from build123d import *

# Parameters (mm, degrees)
SKICA1_W                = 18.57
SKICA1_H                = 8.22
P_IDAT_VYSUNUT_M1_DEPTH = 5
SKICA2_W                = 18.7
SKICA2_H                = 4.88
P_IDAT_VYSUNUT_M2_DEPTH = 28.3
SKICA3_W                = 13.3
SKICA3_H                = 1.1
P_IDAT_VYSUNUT_M3_DEPTH = 5.3


with BuildPart() as part:
    # Skica1 → Přidat vysunutím1 (new body)
    with BuildSketch(Plane.XY):
        Rectangle(SKICA1_W, SKICA1_H)
    extrude(amount=P_IDAT_VYSUNUT_M1_DEPTH)

    # Skica2 → Přidat vysunutím2 (add)
    with BuildSketch(Plane(origin=(0, 4.11, 0), x_dir=(1, 0, 0), z_dir=(0, 1, 0))):
        with Locations((0, -2.5)):
            Rectangle(SKICA2_W, SKICA2_H)
    extrude(amount=P_IDAT_VYSUNUT_M2_DEPTH)

    # Skica3 → Přidat vysunutím3 (add)
    with BuildSketch(Plane(origin=(0, 32.41, 0), x_dir=(1, 0, 0), z_dir=(0, 1, 0))):
        with Locations((0, -4.39)):
            Rectangle(SKICA3_W, SKICA3_H)
    extrude(amount=P_IDAT_VYSUNUT_M3_DEPTH)


solid = part.part
Build history of the part. All positions in model axes, mm. A direction names the side the tool comes from. Coordinates: 2 decimals unless noted, no trailing zeros. Order: outer loops, then holes, each group sorted by start corner. A loop starts at its lowest first (then second) coordinate and runs counter-clockwise, first axis right, second up. Notation, with made-up numbers: (70, 10) - (129, 10) arc R15 cw to (129, 19) - close; hole circle Ø11 at (-12, 16). An arc over 180 degrees is marked (long way). Write item = value, one per line. Start each with the question number.
1) Saw through at A-A on z = 1.1. Write the cut outline in (x, y) (3 decimals), then the cut area to 3 significant figures.
2) Flat gauge pins, fed straight in: pin 1 Ø9.5 at (x, y) = (-4.5, 18) entering from -Z; pin 2 Ø1.2 at (y, z) = (35.5, 4.5) entering from +X; pin 3 Ø2.5 at (x, y) = (3.5, 35) entering from -Z. Where does each tip first touch, or does it go through?
3) Saw through at D-D on z = 4.35. Write the cut outline in (x, y) (3 decimals).
4) Saw through at C-C on y = 6.5. Write the cut outline in (x, z).
5) Saw through at B-B on x = -7.25. Write the cut outline in (y, z).
6) 3-axis set-ups, long thin cutter, end or side, ignore diameter. For faces 1 (the face through (-6.65, 35, 4)), 2 (the face through (6.65, 35, 4)), 3 (the face through (0, 21, 4.94)): which of +Z, -Z, +X, -X, +Y, -Y reach the whole face in a straight line?
7) Wall check: line 1 along Y through (x, z) = (-8, 4.3); line 2 along Z through (x, y) = (-5, 11). Give the ranges that are in metal, low to high. Write a range as from..to.
From the geometry:
q1.outline = (-9.35, 4.11) - (-9.285, 4.11) - (-9.285, -4.11) - (9.285, -4.11) - (9.285, 4.11) - (9.35, 4.11) - (9.35, 32.41) - (-9.35, 32.41) - close
q1.area = 682 mm^2
q2.pin_1 = 0.06
q2.pin_2 = 6.65
q2.pin_3 = 3.84
q3.outline = (-9.35, 4.11) - (-9.285, 4.11) - (-9.285, -4.11) - (9.285, -4.11) - (9.285, 4.11) - (9.35, 4.11) - (9.35, 32.41) - (6.65, 32.41) - (6.65, 37.71) - (-6.65, 37.71) - (-6.65, 32.41) - (-9.35, 32.41) - close
q4.outline = (-9.35, 0.06) - (9.35, 0.06) - (9.35, 4.94) - (-9.35, 4.94) - close
q5.outline = (-4.11, 0) - (4.11, 0) - (4.11, 0.06) - (32.41, 0.06) - (32.41, 4.94) - (4.11, 4.94) - (4.11, 5) - (-4.11, 5) - close
q6.face_1 = +Z, -Z, -X, +Y
q6.face_2 = +Z, -Z, +X, +Y
q6.face_3 = +Z, +X, -X, +Y
q7.line_1 = -4.11..32.41
q7.line_2 = 0.06..4.94
